Job drawing, mm, ordinate dimensions from the low corner. One solid piece. A direction names the side the tool comes from. Coordinates: 2 decimals unless noted, no trailing zeros. Use a Markdown table: item, result. Add a question column.
1. 3-axis set-ups, long thin cutter, end or side, ignore diameter. For the marked faces 1 and 2: which of +Z, -Z, +X, -X, +Y, -Y reach the whole face in a straight line?
2. Band-saw the part on D-D, the plane z = 29.5. Count the separate pieces of the cut face and the enclosed holes in it, plus the area to 3 significant figures.
3. Wall check: probe 1 along Z at (x, y) = (14, 78) (1 decimal); probe 2 along Z at (x, y) = (7, 80.5) (1 decimal). Give the ranges that are in metal, low to high. Write a range as [from, to].
4. Drop flat-ended pins along their axis: pin 1 (19 mm diameter, centred on x = 23, y = 52.5, fed in from -Z) (1 decimal); pin 2 (11.5 mm diameter, centred on x = 26.99, y = 20.64, fed in from +Z). Give the stop position or say it passes through.
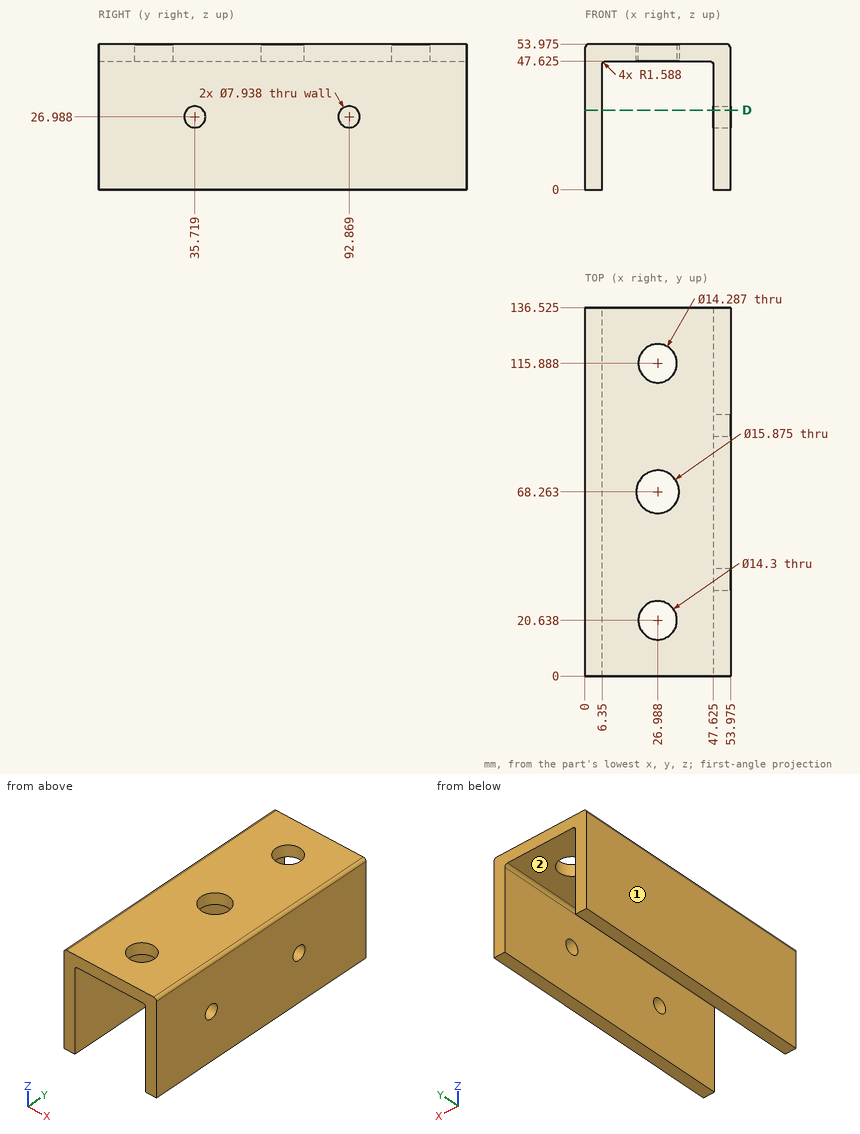
Geometry check:
| question | item | result |
|---|---|---|
| 1 | face 1 | +Z, -Z, -X, +Y, -Y |
| 1 | face 2 | -Z, +Y, -Y |
| 2 | separate pieces | 4 |
| 2 | enclosed holes | 0 |
| 2 | area | 1,660 mm^2 |
| 3 | probe 1 | z = [47.6, 54] |
| 3 | probe 2 | z = [47.3, 54] |
| 4 | pin 1 | stops at z = 47.6 |
| 4 | pin 2 | passes through |
